from build123d import *

# Parameters (mm, degrees)
BOSS_EXTRUDE1_DEPTH      = 12
BOSS_EXTRUDE1_DEPTH_BACK = 2
SCALE1_SCALE             = 0.184184676
CUT_EXTRUDE1_REACH       = 177.722
SKETCH4_R                = 2.5


with BuildPart() as part:
    # Sketch3 → Boss-Extrude1 (new, two sides: drawn at the far end of the back side and taken through both)
    with BuildSketch(Plane(origin=(0, 0, 0), x_dir=(0, 0, -1), z_dir=(1, 0, 0)).offset(-BOSS_EXTRUDE1_DEPTH_BACK)):
        with BuildLine():
            Line((0, -60), (0, -86.184781703))
            ThreePointArc((0, -86.184781703), (14.644660941, -121.540120762), (50, -136.184781703))
            Line((50, -136.184781703), (59.297038535, -136.184781703))
            ThreePointArc((59.297038535, -136.184781703), (94.227856727, -150.409958986), (109.282791662, -184.991264087))
            Line((109.282791662, -184.991264087), (110.272400942, -226.437125049))
            ThreePointArc((110.272400942, -226.437125049), (107.627548101, -240.207635718), (95.065077273, -246.437125049))
            Line((95.065077273, -246.437125049), (72.641071037, -246.437125049))
            ThreePointArc((72.641071037, -246.437125049), (62.034469319, -250.830523332), (57.641071037, -261.437125049))
            Line((57.641071037, -261.437125049), (57.641071037, -278.751269833))
            ThreePointArc((57.641071037, -278.751269833), (60.570003225, -285.822337645), (67.641071037, -288.751269833))
            Line((67.641071037, -288.751269833), (116.127942723, -288.751269833))
            Line((116.127942723, -288.751269833), (138.939006392, -288.751269833))
            ThreePointArc((138.939006392, -288.751269833), (153.081142016, -282.893405456), (158.939006392, -268.751269833))
            Line((158.939006392, -268.751269833), (158.939006392, -146.184781703))
            Line((158.939006392, -146.184781703), (158.939006392, -50))
            Line((158.939006392, -50), (158.939006392, -11.480346054))
            ThreePointArc((158.939006392, -11.480346054), (148.053108697, 21.328755123), (117.156078712, 36.830801017))
            ThreePointArc((117.156078712, 36.830801017), (39.60735059, 11.368133348), (0, -60))
        make_face()
    extrude(amount=BOSS_EXTRUDE1_DEPTH + BOSS_EXTRUDE1_DEPTH_BACK)


with BuildPart() as part_1:
    # Scale1: scaled about (5, -104.808897059, -96.321000263)
    add(part.part.scale(SCALE1_SCALE).moved(Location((4.07907662, -85.504704312, -78.580148038))))

    # Sketch4 → Cut-Extrude1 (cut, up to next)
    with BuildSketch(Plane(origin=(6.289292732, 0, 0), x_dir=(0, 0, -1), z_dir=(1, 0, 0)), mode=Mode.PRIVATE) as cut_extrude1_sk1:
        with Locations((95.143312613, -96.09592734)):
            Circle(SKETCH4_R)
    cut_extrude1_tool1 = extrude(cut_extrude1_sk1.sketch, amount=-CUT_EXTRUDE1_REACH, mode=Mode.PRIVATE) & part_1.part
    add(cut_extrude1_tool1.solids().sort_by_distance((6.289293, -96.095927, -95.143313))[0], mode=Mode.SUBTRACT)


solid = part_1.part
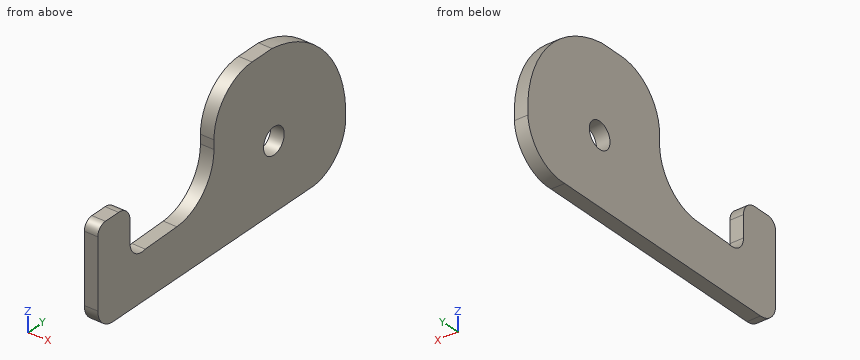
Design review of the part built by this model. Coordinates are the model's own, in mm. Give positions to 0.01 mm unless a question says otherwise; leave off trailing zeros. Order: outer loops, then holes, each group sorted by start corner. A loop starts at its lowest first (then second) coordinate and runs counter-clockwise, first axis right, second up. Notation, with made-up numbers: (19, 22.25) - (57, 22.25) arc R18 cw to (57, 53.25) - close; hole circle Ø11 at (45, -32). An arc over 180 degrees is marked (long way). Write item = value, one per line. Start each with the question number.
Q1. We need section A-A on z = -93.75. State the section outline as (x, y) points.
Q2. We need section D-D on x = 4.2. State the section outline as (y, z) points.
Q3. We need section B-B on y = -95.5. State the section outline as (x, z) points, plus the area to 3 significant figures.
Q4. To check wall thickness, follow L1, parallel to Y at x = 4.45, z = -94; L2, parallel to Y at x = 5.2, z = -94.5; L3, parallel to Y at x = 5.5, z = -92. State the ranges of each line that lie inside material, in increasing order. Write a range as from..to.
Q5. We need section C-C on z = -90.5. State the section outline as (x, y) points, plus the area to 3 significant figures.
Q6. Clearance check with flat-ended pins moving along their axes: pin 1 Ø1.3 at (x, y) = (4.5, -134.5) entering from +Z; pin 2 Ø0.9 at (x, z) = (5, -88.5) entering from -Y. State where each tip first meets the part, or that it passes through.
Working result:
q1.outline = (3.71, -138.69) - (6.29, -138.69) - (6.29, -130.89) - (3.71, -130.89) - close; (3.71, -111.63) - (6.29, -111.63) - (6.29, -98.17) - (3.71, -98.17) - close; (3.71, -94.02) - (6.29, -94.02) - (6.29, -79.37) - (3.71, -79.37) - close
q2.outline = (-138.69, -104.17) arc R3.68 ccw to (-135, -107.85) - (-87.62, -107.85) arc R8.32 ccw to (-78.72, -100.16) arc R20.6 ccw to (-96.56, -78.58) - (-101.38, -78.58) arc R9.21 ccw to (-110.59, -87.79) - (-110.59, -89.5) arc R9.21 cw to (-119.58, -98.71) - (-127.21, -98.89) arc R2.91 cw to (-130.89, -96.09) - (-130.89, -91.96) arc R2.76 ccw to (-133.66, -89.2) - (-136.85, -89.2) arc R1.84 ccw to (-138.69, -91.04) - close; hole circle Ø5 at (-96.1, -95.14)
q3.outline = (3.71, -107.85) - (6.29, -107.85) - (6.29, -97.57) - (3.71, -97.57) - close; (3.71, -92.72) - (6.29, -92.72) - (6.29, -78.75) - (3.71, -78.75) - close
q3.area = 62.5 mm²
q4.L1 = -138.69..-130.89, -111.76..-98.32, -93.87..-79.3
q4.L2 = -138.69..-130.89, -112.06..-98.51, -93.68..-79.19
q4.L3 = -138.69..-130.89, -110.93..-79.91
q5.outline = (3.71, -138.61) - (6.29, -138.61) - (6.29, -131.31) - (3.71, -131.31) - close; (3.71, -110.64) - (6.29, -110.64) - (6.29, -80.52) - (3.71, -80.52) - close
q5.area = 96.5 mm²
q6.pin_1 = -89.2
q6.pin_2 = -110.59
